Autodesk Inventor part; units mm, degrees
ref_plane "YZ Plane" through (0, 0, 0) normal (1, 0, 0) x (0, 1, 0)
ref_plane "XZ Plane" through (0, 0, 0) normal (0, 1, 0) x (-1, 0, 0)
ref_plane "XY Plane" through (0, 0, 0) normal (0, 0, 1) x (1, 0, 0)
sketch "Sketch1" plane through (0, 0, 0) normal (0, 0, 1) x (1, 0, 0)
  circle A0 centre (0, 0) radius 2
  line L0 (-4.5, 4) -> (4.5, 4)
  line L1 (4.5, 4) -> (4.5, -4)
  line L2 (4.5, -4) -> (-4.5, -4)
  line L3 (-4.5, -4) -> (-4.5, 4)
  line L4 (-4.5, 4) -> (4.5, -4) construction
  dimension "d0" = 4
  dimension "d1" = 8
  dimension "d2" = 9
extrude "Plate1" add sketch "Sketch1" along normal blind 0.8
sketch "Sketch2" plane through (3.7, 4, 0) normal (1, 0, 0) x (0, 1, 0)
  line L0 (-8, 0) -> (0, 0)
  line L1 (0, 0) -> (0, 15)
  line L2 (0, 15) -> (-8, 15)
  line L3 (-8, 15) -> (-8, 0)
edge flange "Flange1" height 15 angle 90 thickness 0.8 bend radius 0.8 thickness toward (1, 0, 0) relief tear relief width 0.8 relief depth 0.4 corner gap 0.8 corner form 0 edges at (4.5, 0, 0.8) (-4.5, 0, 0.8) wall of the first edge with corners at (3.7, -4, 0) (3.7, 4, 0) (3.7, 4, 15) (3.7, -4, 15)
bend "Bend1"
corner "Corner1"
sketch "Sketch3" plane through (-4.5, -4, 15) normal (-1, 0, 0) x (0, 0, 1)
  line L0 (-13.4, 8) -> (-13.4, 0) construction
  line L1 (0, 0) -> (-13.4, 0)
  line L2 (0, 8) -> (0, 0)
  line L3 (-13.4, 8) -> (0, 8)
  circle A0 centre (-4, 4) radius 4
  point P0 (-15, 4)
  point P1 (-4, 8)
  point P2 (0, 4)
  point P3 (-4, 0)
extrude "Cut1" cut sketch "Sketch3" against normal through all contours L1 A0 L2 | A0 L3 L2
sketch "Sketch4" plane through (-4.5, -4, 1.6) normal (-1, 0, 0) x (0, 0, 1)
  arc A0 (9.4, 0) -> (9.4, 8) centre (9.4, 4) ccw
  circle A1 centre (9.4, 4) radius 2
  point P0 (-1.6, 4)
  dimension "d16" = 4
extrude "Cut2" cut sketch "Sketch4" against normal through all
equation "\"d14\" = Thickness"
equation "\"d17\" = Thickness"
equation "\"d3\" = Thickness"
equation "\"d4\" = BendReliefWidth"
equation "\"d5\" = BendReliefDepth"
equation "\"d6\" = MinimumRemnant"
equation "\"d7\" = TransitionRadius"
equation "\"d10\" = BendRadius"
equation "\"d11\" = CornerReliefSize"
equation "\"d12\" = GapSize"
equation "\"d13\" = JacobiRadiusSize"
equation "\"BendRadius\" = Thickness"
equation "\"BendReliefWidth\" = Thickness"
equation "\"BendReliefDepth\" = 0.5 * Thickness"
equation "\"CornerReliefSize\" = 4 * Thickness"
equation "\"MinimumRemnant\" = 2 * Thickness"
equation "\"TransitionRadius\" = BendRadius"
equation "\"JacobiRadiusSize\" = BendRadius"
equation "\"GapSize\" = Thickness"
properties part number "LA-T8-Bracket"
Part model, mm, in its own coordinate system. A direction names the side the tool comes from. Coordinates: 2 decimals unless noted, no trailing zeros. Order: outer loops, then holes, each group sorted by start corner. A loop starts at its lowest first (then second) coordinate and runs counter-clockwise, first axis right, second up. Notation, with made-up numbers: (-6.75, 54.5) - (4.25, 54.5) arc R26 ccw to (4.25, 75.5) - close; hole circle Ø2 at (1.25, 59). An arc over 180 degrees is marked (long way). Return JSON: item names as keys, results as strings. Group by question number.
Item 1: Drill centre lines: probe 1 along Y at (x, z) = (-4.15, 11); probe 2 along X at (y, z) = (-2.5, 8.75); probe 3 along Z at (x, y) = (-2.5, -0.25). Where is each one in solid material? Low to high. Write a range as from..to.
Item 2: Cut at A-A (y = 0). List the corners of the cut face in (x, z), plus the area to 3 significant figures.
Item 3: Pull direction Y, two halves, no side cores. Call faces 3 (the face through (4, 0, 15)), 4 (the face through (-4.04, -0.06, 0.48)), 5 (the face through (4.1, -1.2, 9.4)): pulls with the +Y half, pulls with the -Y half, needs draft (parallel to the pull), parting line crosses it, or undercut.
Item 4: Which spindle directions (+Z, -Z, +X, -X, +Y, -Y) get a long thin tool onto all of the face, cutting with end or side? Do faces 1 (the face through (4.04, 0.06, 0.48)), 2 (the face through (3.47, 0.06, 1.04)). Say none if no direction does.
Item 5: Cut at D-D (x = 4). List the corners of the cut face in (y, z).
Item 6: Pin check, flat tips, straight feed: pin 1 (4.5 mm diameter, centred on x = 0, y = 0, fed in from +Z); pin 2 (2.5 mm diameter, centred on y = 0, z = 11, fed in from +X). Stop position of each tip, or through.
Item 7: Cut at B-B (z = 8). List the corners of the cut face in (x, y).
Item 8: Cut at C-C (x = 0). List the corners of the cut face in (y, z).
Check values:
{
 "1": {"probe 1": "y = -4..-2, 2..4", "probe 2": "x = -4.5..-3.7, 3.7..4.5", "probe 3": "z = 0..0.8"},
 "2": {"outline": "(-4.5, 1.6) arc R1.6 ccw to (-2.9, 0) - (-2, 0) - (-2, 0.8) - (-2.9, 0.8) arc R0.8 cw to (-3.7, 1.6) - (-3.7, 9) - (-4.5, 9) - close; (-4.5, 13) - (-3.7, 13) - (-3.7, 15) - (-4.5, 15) - close; (2, 0) - (2.9, 0) arc R1.6 ccw to (4.5, 1.6) - (4.5, 9) - (3.7, 9) - (3.7, 1.6) arc R0.8 cw to (2.9, 0.8) - (2, 0.8) - close; (3.7, 13) - (4.5, 13) - (4.5, 15) - (3.7, 15) - close", "area": "19.5 mm2"},
 "3": {"face 3": "parting line crosses it", "face 4": "needs draft", "face 5": "undercut"},
 "4": {"face 1": "-Z, +X, +Y, -Y", "face 2": "+Z, +Y, -Y"},
 "5": {"outline": "(-4, 0.44) - (4, 0.44) - (4, 11) arc R4 ccw to (-4, 11) - close; hole circle Ø4 at (0, 11)"},
 "6": {"pin 1": "stops at z = 0.8", "pin 2": "passes through"},
 "7": {"outline": "(-4.5, -4) - (-3.7, -4) - (-3.7, 4) - (-4.5, 4) - close; (3.7, -4) - (4.5, -4) - (4.5, 4) - (3.7, 4) - close"},
 "8": {"outline": "(-4, 0) - (-2, 0) - (-2, 0.8) - (-4, 0.8) - close; (2, 0) - (4, 0) - (4, 0.8) - (2, 0.8) - close"}
}
